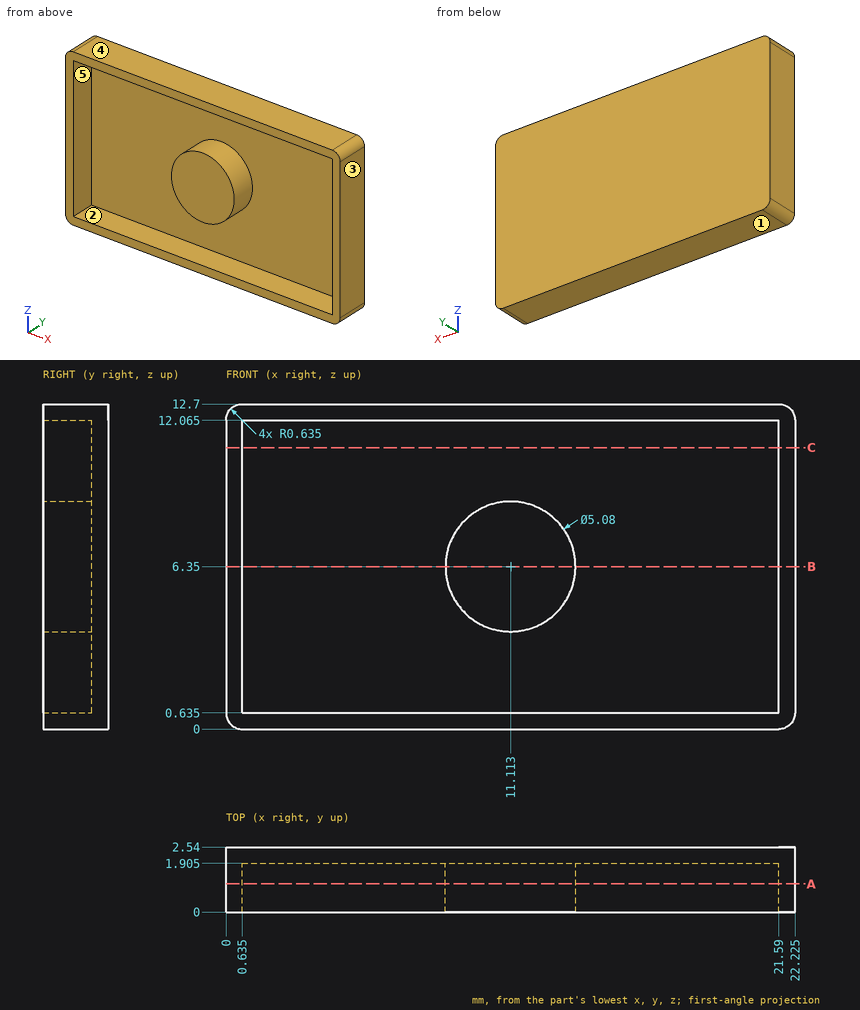
Check sheet for the drawn part. Datum: minimum x, y, z corner. Units: mm. A direction names the side the tool comes from. Round coordinates to 2 decimals unless told otherwise and drop trailing zeros. Loops run counter-clockwise (first coordinate to the right, second up) from the corner with the lowest first, then second, coordinate; pieces in that order, holes last. Notation, with made-up numbers: (-1, 43.5) - (22, 43.5) arc R18 cw to (22, 72.5) - close; hole circle Ø8 at (8.5, -3). An arc over 180 degrees is marked (long way). Answer as a JSON object with one key per item and string values. Group by question number.
Q1. Set-up check for the marked faces 4 and 5: record each of +Z, -Z, +X, -X, +Y, -Y from which the full face is reachable in a straight line by a thin tool's end or side.
Q2. Mould release check, pull along Z, two halves, no side actions. Record for the marked faces 1, 2 and 3: released by +Z, released by -Z, zero draft, split by the parting line, or undercut.
Q3. Sectioned sample at C-C, the plane z = 11. Enter the section's corners in (x, y) (1 decimal).
Q4. Sectioned sample at A-A, the plane y = 1.1. Count the separate pieces of the cut face and the enclosed holes in it.
Q5. Gauge pin test, flat end, axial feed: P1, Ø3.5, axis at x = 16.5, z = 5, coming from the -Y side (1 decimal). Record the tip position at first contact, or that the pin passes through.
Q6. Scan lines: line 1 along Z through (x, y) = (11, 0.35) (1 decimal); line 2 along Z through (x, y) = (16, 0.25) (1 decimal); line 3 along X through (y, z) = (0.55, 11.75) (1 decimal). Record each from-to range of solid material in increasing order. Write a range as [from, to].
Q7. Sectioned sample at B-B, the plane z = 6.35. Enter the section's corners in (x, y) (1 decimal).
Solution:
{
 "1": {"face 4": "+Z, +X, -X, +Y, -Y", "face 5": "-Y"},
 "2": {"face 1": "released by -Z", "face 2": "undercut", "face 3": "zero draft"},
 "3": {"outline": "(0, 0) - (0.6, 0) - (0.6, 1.9) - (21.6, 1.9) - (21.6, 0) - (22.2, 0) - (22.2, 2.5) - (0, 2.5) - close"},
 "4": {"separate pieces": "2", "enclosed holes": "1"},
 "5": {"P1": "stops at y = 1.9"},
 "6": {"line 1": "z = [0, 0.6], [3.8, 8.9], [12.1, 12.7]", "line 2": "z = [0, 0.6], [12.1, 12.7]", "line 3": "x = [0, 0.6], [21.6, 22.2]"},
 "7": {"outline": "(0, 0) - (0.6, 0) - (0.6, 1.9) - (8.6, 1.9) - (8.6, 0) - (13.7, 0) - (13.7, 1.9) - (21.6, 1.9) - (21.6, 0) - (22.2, 0) - (22.2, 2.5) - (0, 2.5) - close"}
}
